from build123d import *

# Parameters (mm, degrees)
F0_R     = 10
F1_DEPTH = 8


with BuildPart() as f1:
    # F0 (on Top) → F1 (new body)
    with BuildSketch(Plane.XY):
        with BuildLine():
            ThreePointArc((-2, 0), (-0.585786, -0.585786), (0, -2))
            Line((0, -2), (0, -39.817824))
            ThreePointArc((0, -39.817824), (1.279892, -41.683687), (3.481445, -41.161447))
            Line((3.481445, -41.161447), (40.813559, 0))
            Line((40.813559, 0), (130.9251, 95.263347))
            Line((130.9251, 95.263347), (142.5, 107.5))
            Line((142.5, 107.5), (142.5, 125))
            Line((142.5, 125), (142.5, 135))
            ThreePointArc((142.5, 135), (140.303301, 140.303301), (135, 142.5))
            Line((135, 142.5), (116.793654, 142.5))
            Line((116.793654, 142.5), (104.779634, 129.799121))
            Line((104.779634, 129.799121), (-18, 0))
            Line((-18, 0), (-18, -44.289797))
            ThreePointArc((-18, -44.289797), (-17.314199, -44.81378), (-16.471463, -45))
            Line((-16.471463, -45), (-11, -45))
            ThreePointArc((-11, -45), (-9.585786, -44.414214), (-9, -43))
            Line((-9, -43), (-9, -2))
            ThreePointArc((-9, -2), (-8.414214, -0.585786), (-7, 0))
            Line((-7, 0), (-2, 0))
        make_face()
        with BuildLine():
            Line((34.354794, 7.5), (16.836377, 7.5))
            ThreePointArc((16.836377, 7.5), (9.94782, 12.033895), (11.387794, 20.153925))
            Line((11.387794, 20.153925), (51.345731, 62.396315))
            ThreePointArc((51.345731, 62.396315), (56.501034, 64.736653), (61.823464, 62.80635))
            Line((61.823464, 62.80635), (71.310982, 54.230777))
            ThreePointArc((71.310982, 54.230777), (73.77628, 48.955349), (71.723881, 43.505992))
            Line((71.723881, 43.505992), (39.803376, 9.846075))
            ThreePointArc((39.803376, 9.846075), (37.320899, 8.111443), (34.354794, 7.5))
        make_face(mode=Mode.SUBTRACT)
        with BuildLine():
            ThreePointArc((120.047881, 105.578456), (122.384292, 100.340012), (120.335639, 94.982482))
            Line((120.335639, 94.982482), (86.723895, 59.449106))
            ThreePointArc((86.723895, 59.449106), (81.483666, 57.105926), (76.121387, 59.154449))
            Line((76.121387, 59.154449), (66.875695, 67.900137))
            ThreePointArc((66.875695, 67.900137), (64.532515, 73.140366), (66.581038, 78.502645))
            Line((66.581038, 78.502645), (100.203863, 114.047735))
            ThreePointArc((100.203863, 114.047735), (105.448841, 116.391046), (110.81327, 114.335858))
            Line((110.81327, 114.335858), (120.047881, 105.578456))
        make_face(mode=Mode.SUBTRACT)
        with Locations((125, 125)):
            Circle(F0_R, mode=Mode.SUBTRACT)
    extrude(amount=F1_DEPTH)


solid = f1.part
For this review, take the finished solid that the model builds, in its own axes (mm). A direction names the side the tool comes from. Give positions to 0.01 mm unless a question says otherwise; leave off trailing zeros. Loops run counter-clockwise (first coordinate to the right, second up) from the corner with the lowest first, then second, coordinate; pieces in that order, holes last. Notation, with made-up numbers: (78.5, 21) -> (127.5, 21) arc R17 cw to (127.5, 46) -> close; hole circle Ø2 at (79.5, 9.25). An arc over 180 degrees is marked (long way). One line per question, with ' | ' between items.
1) For faces 4 (the flat face through (44, 56, 8)), 5 (the flat face through (31.09, 40.98, 3.94)), 6 (the flat face through (-5, 0, 4)), list the 3-axis set-ups (+Z, -Z, +X, -X, +Y, -Y) from which the entire face can be reached by the end or side of a thin tool; tool diameter is ignored.
Resolved:
face 4: +Z, +X, -X, +Y, -Y | face 5: +Z, -Z | face 6: +Z, -Z, -Y
2) We need section B-B (y = 110.5). Write out the cut boundary in (x, z).
Resolved:
outline: (86.52, 0) -> (96.85, 0) -> (96.85, 8) -> (86.52, 8) -> close; (114.86, 0) -> (142.5, 0) -> (142.5, 8) -> (114.86, 8) -> close
3) To check wall thickness, follow probe 1 along X at (y, z) = (-4, 1.25); probe 2 along Y at (x, z) = (125, 6.25); probe 3 along X at (y, z) = (15.5, 3.75). State the ranges of each line that lie inside material, in increasing order.
Resolved:
probe 1: x = -18 to -9, 0 to 37.19 | probe 2: y = 89 to 115, 135 to 142.5 | probe 3: x = -3.34 to 9.35, 45.17 to 55.48
4) Insertion check: pin 1 Ø1.5 at (x, z) = (98, 7) entering from +Y; pin 2 Ø2 at (x, z) = (78, 4) entering from +Y; pin 3 Ø1.5 at (x, z) = (-4, 2.5) entering from -Y. Each pin has a flat end and moves straight along its axis. Give the tip position at first contact, or say it passes through.
Resolved:
pin 1: stops at y = 123.42 | pin 2: stops at y = 102.55 | pin 3: stops at y = 0
5) We need section A-A (x = 107). Write out the cut boundary in (y, z), plus the area to 3 significant figures.
Resolved:
outline: (69.97, 0) -> (80.88, 0) -> (80.88, 8) -> (69.97, 8) -> close; (116.27, 0) -> (132.15, 0) -> (132.15, 8) -> (116.27, 8) -> close | area: 214 mm2
6) The part is to be moulded in two halves that separate along X. For faces 1 (the flat face through (115.366, 110.018, 3.944)), 2 (the flat face through (44, 56, 0)), 3 (the flat face through (21.886, -20.869, 3.944)), say which applies: +X half, -X half, draft (parallel to the pull), parting line (faces both ways), or undercut.
Resolved:
face 1: undercut | face 2: draft | face 3: +X half
7) We need section C-C (z = 5.25). Give the number of separate pieces and of enclosed holes in the cut face, plus the area to 3 significant figures.
Resolved:
separate pieces: 1 | enclosed holes: 3 | area: 5,210 mm2
